Source: CAD feature listing. Evaluate the final solid. Frame: model axes, mm. A direction names the side the tool comes from. Round coordinates to 2 decimals unless told otherwise and drop trailing zeros. Order: outer loops, then holes, each group sorted by start corner. A loop starts at its lowest first (then second) coordinate and runs counter-clockwise, first axis right, second up. Notation, with made-up numbers: (68.25, -7.75) -> (124.25, -7.75) arc R22 cw to (124.25, 23.25) -> close; hole circle Ø5 at (44.5, 49). An arc over 180 degrees is marked (long way). One line per item, written item: value. Start each with the question number.
1) Mould query, pull axis X, two halves, no side actions, for faces 4 (the face through (273, 1, 0)), 5 (the face through (254.7, 57, 3)), 6 (the face through (271.756, -30.986, 3.131)). Classes: pulls with the +X half, pulls with the -X half, needs draft (parallel to the pull), parting line crosses it, or undercut.
2) Pin query (flat end, axial travel): P1, Ø3, axis at y = -21.5, z = 4.5, coming from the -X side. Return the tip coordinate at first contact, or that it passes through.
3) Section A-A (x = 259). Return the cut outline in (y, z), and give its area (3 significant figures).
4) Ray query, L1, parallel to Y at x = 266, z = 3; L2, parallel to Y at x = 277, z = 3.5; L3, parallel to X at y = -23.5, z = 1.5. Return the intervals inside material, ascending.
5) Section B-B (z = 1). Return the cut outline in (x, y).
6) Reachability of faces 1 (the face through (278.7, 19, 3)), 2 (the face through (273, -82.55, 3)), 3 (the face through (264, -31.75, 3)) from +Z, -Z, +X, -X, +Y, -Y: full face, straight path, thin tool, end or side. Return the list, or none.
Autodesk Inventor part; units mm, degrees
ref_plane "YZ Plane" through (0, 0, 0) normal (1, 0, 0) x (0, 1, 0)
ref_plane "XZ Plane" through (0, 0, 0) normal (0, 1, 0) x (-1, 0, 0)
ref_plane "XY Plane" through (0, 0, 0) normal (0, 0, 1) x (1, 0, 0)
ref_plane "Work Plane1" through (0, 0, 0) normal (0, 0, 1) x (1, 0, 0)
sketch "Sketch1" plane through (0, 0, 0) normal (0, 0, 1) x (1, 0, 0)
  line L0 (254.7, -154.94) -> (254.7, 140.97)
  line L1 (291.2125, 168.0875) -> (291.2125, -168.0875)
  arc A0 (256.7, 31.75) -> (254.7, 29.75) centre (256.7, 29.75) ccw
  line L2 (254.7, 29.75) -> (254.7, 8.75)
  arc A1 (254.7, 8.75) -> (256.7, 6.75) centre (256.7, 8.75) ccw
  line L3 (256.7, 6.75) -> (276.7, 6.75)
  arc A2 (276.7, 6.75) -> (278.7, 8.75) centre (276.7, 8.75) ccw
  line L4 (278.7, 8.75) -> (278.7, 29.75)
  arc A3 (278.7, 29.75) -> (276.7, 31.75) centre (276.7, 29.75) ccw
  line L5 (276.7, 31.75) -> (256.7, 31.75)
  circle A4 centre (276.78, 8.75) radius 1.05
  circle A5 centre (264.2, 8.75) radius 1.05
  circle A6 centre (276.78, 29.75) radius 1.05
  circle A7 centre (264.2, 29.75) radius 1.05
  arc A8 (257.24, -13.97) -> (254.7, -16.51) centre (257.24, -16.51) ccw
  line L6 (254.7, -16.51) -> (254.7, -29.21)
  arc A9 (254.7, -29.21) -> (257.24, -31.75) centre (257.24, -29.21) ccw
  line L7 (257.24, -31.75) -> (269.94, -31.75)
  arc A10 (269.94, -31.75) -> (272.48, -29.21) centre (269.94, -29.21) ccw
  line L8 (272.48, -29.21) -> (272.48, -16.51)
  arc A11 (272.48, -16.51) -> (269.94, -13.97) centre (269.94, -16.51) ccw
  line L9 (269.94, -13.97) -> (257.24, -13.97)
  circle A12 centre (257.24, -19.05) radius 0.5
  circle A13 centre (257.24, -24.13) radius 0.5
  circle A14 centre (257.24, -29.21) radius 0.5
  circle A15 centre (269.94, -29.21) radius 1.25
  circle A16 centre (259.272, -18.923) radius 0.25
  circle A17 centre (269.178, -19.304) radius 0.25
  circle A18 centre (263.463, -28.702) radius 0.25
  circle A19 centre (268.289, -26.67) radius 0.25
  circle A20 centre (267.654, -30.861) radius 0.25
  circle A21 centre (260.669, -26.797) radius 0.25
  circle A22 centre (265.622, -26.035) radius 0.25
  circle A23 centre (267.654, -21.717) radius 0.25
  circle A24 centre (260.796, -21.971) radius 0.25
  circle A25 centre (269.94, -16.51) radius 1.25
  circle A26 centre (257.24, -26.67) radius 0.5
  circle A27 centre (257.24, -21.59) radius 0.5
  circle A28 centre (257.24, -16.51) radius 0.5
  line L10 (254.7, 31.75) -> (254.7, 82.55)
  line L11 (254.7, 82.55) -> (291.2125, 82.55)
  line L12 (254.7, 31.75) -> (256.7, 31.75)
  line L13 (256.7, 6.75) -> (254.7, 6.75)
  line L14 (257.24, -13.97) -> (254.7, -13.97)
  line L15 (257.175, -31.75) -> (254.7, -31.75)
  line L16 (254.7, -31.75) -> (254.7, -82.55)
  line L17 (254.7, -82.55) -> (291.2125, -82.55)
  point P0 (0, 0)
  dimension "d0" = 50.8
  dimension "d1" = 50.8
extrude "Extrusion1" add sketch "Sketch1" along normal blind 6.35 contours L0 L15 A9 L7 A10 L8 A11 L9 L14 L13 L3 A2 L4 A3 L5 L12 L11 L1 L17 | L0 A9 L15
Findings:
1. face 4: needs draft
1. face 5: pulls with the -X half
1. face 6: undercut
2. P1: x = 272.48
3. outline: (-82.55, 0) -> (-31.75, 0) -> (-31.75, 6.35) -> (-82.55, 6.35) -> close; (-13.97, 0) -> (6.75, 0) -> (6.75, 6.35) -> (-13.97, 6.35) -> close; (31.75, 0) -> (82.55, 0) -> (82.55, 6.35) -> (31.75, 6.35) -> close
3. area: 777 mm2
4. L1: -82.55 to -31.75, -13.97 to 6.75, 31.75 to 82.55
4. L2: -82.55 to 6.77, 31.73 to 82.55
4. L3: 272.48 to 291.21
5. outline: (254.7, -82.55) -> (291.21, -82.55) -> (291.21, 82.55) -> (254.7, 82.55) -> (254.7, 31.75) -> (276.7, 31.75) arc R2 cw to (278.7, 29.75) -> (278.7, 8.75) arc R2 cw to (276.7, 6.75) -> (254.7, 6.75) -> (254.7, -13.97) -> (269.94, -13.97) arc R2.54 cw to (272.48, -16.51) -> (272.48, -29.21) arc R2.54 cw to (269.94, -31.75) -> (257.24, -31.75) arc R2.54 cw to (254.7, -29.21) -> close
6. face 1: +Z, -Z, -X
6. face 2: +Z, -Z, +X, -X, -Y
6. face 3: +Z, -Z
